Part print with two shaded views. Sizes in mm from the minimum x, y, z corner. A direction names the side the tool comes from. Give positions to 0.01 mm unless a question says otherwise; leave off trailing zeros. Order: outer loops, then holes, each group sorted by start corner. A loop starts at its lowest first (then second) coordinate and runs counter-clockwise, first axis right, second up. Notation, with made-up numbers: M -19.5,-31 L 13.5,-31 A18 ccw 13.5,2 Z; hole C -5.5,-34 d6. An arc over 180 degrees is marked long. Return JSON: item names as keys, results as strings. Group by question number.
1. Slice it at B-B on y = 8.5. List the corners of the cut face in (x, z).
2. Pin check, flat tips, straight feed: pin 1 (3 mm diameter, centred on x = 59.5, z = 7, fed in from -Y); pin 2 (5 mm diameter, centred on x = 35, y = 7.5, fed in from +Z). Stop position of each tip, or through.
3. 3-axis set-ups, long thin cutter, end or side, ignore diameter. For the marked faces 1, 2 and 3: which of +Z, -Z, +X, -X, +Y, -Y reach the whole face in a straight line?
4. Wall check: probe 1 along X at (y, z) = (9.25, 3.5); probe 2 along Z at (x, y) = (29, 3); probe 3 along X at (y, z) = (15.25, 4). Give the ranges that are in metal, low to high. Write a range as [from, to].
5. Slice it at D-D on x = 28.5. List the corners of the cut face in (y, z), then the cut area to 3 significant figures.
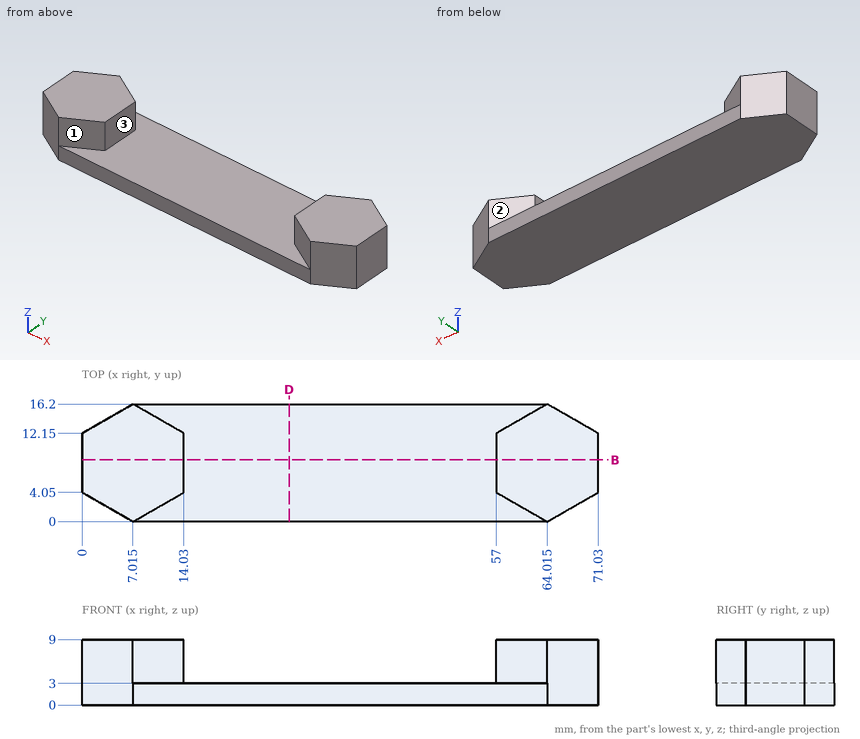
Result:
{
 "1": {"outline": "M 0,0 L 71.03,0 L 71.03,9 L 57,9 L 57,3 L 14.03,3 L 14.03,9 L 0,9 Z"},
 "2": {"pin 1": "stops at y = 1.74", "pin 2": "stops at z = 3"},
 "3": {"face 1": "+Z, -Y", "face 2": "+Z, +Y", "face 3": "+Z, +Y, -Y"},
 "4": {"probe 1": "x = [0, 14.03], [57, 71.03]", "probe 2": "z = [0, 3]", "probe 3": "x = [5.37, 8.66], [62.37, 65.66]"},
 "5": {"outline": "M 0,0 L 16.2,0 L 16.2,3 L 0,3 Z", "area": "48.6 mm2"}
}
